Design review of the part built by this model. Coordinates are the model's own, in mm. A direction names the side the tool comes from. Coordinates: 2 decimals unless noted, no trailing zeros. Order: outer loops, then holes, each group sorted by start corner. A loop starts at its lowest first (then second) coordinate and runs counter-clockwise, first axis right, second up. Notation, with made-up numbers: M 41,54.5 L 59,54.5 A12 cw 59,63.5 Z; hole C 81,38 d1. An arc over 180 degrees is marked long. Answer in a Markdown table with one row per item.
Autodesk Fusion 360 part; units mm, degrees
sketch "Sketch1" plane through (0, 0, 0) normal (0, 1, 0) x (1, 0, 0)
  line L0 (55, -90) -> (-55, -90)
  line L1 (-55, -90) -> (-55, 90)
  line L2 (-55, 90) -> (55, 90)
  line L3 (55, 90) -> (55, -90)
  line L4 (55, -90) -> (-55, 90) construction
  line L5 (-55, -90) -> (55, 90) construction
  dimension "d1" = 180
  dimension "d2" = 110
extrude "Extrude1" add sketch "Sketch1" along normal blind 50
sketch "Sketch2" plane through (0, 50, 0) normal (0, 1, 0) x (-1, 0, 0)
  line L0 (-55, -90) -> (55, -90)
  line L1 (55, -90) -> (55, 90)
  line L2 (55, 90) -> (-55, 90)
  line L3 (-55, 90) -> (-55, -90)
  line L4 (55, -90) -> (30, -90)
  line L5 (30, -90) -> (30, -40)
  line L6 (30, -40) -> (55, -40)
  line L7 (55, -40) -> (55, -90)
  line L8 (30, -90) -> (10, -90)
  line L9 (10, -90) -> (10, -40)
  line L10 (10, -40) -> (30, -40)
  line L11 (30, -40) -> (30, -90)
  line L12 (10, -90) -> (-10, -90)
  line L13 (-10, -90) -> (-10, -40)
  line L14 (-10, -40) -> (10, -40)
  line L15 (10, -40) -> (10, -90)
  line L16 (-10, -90) -> (-30, -90)
  line L17 (-30, -90) -> (-30, -40)
  line L18 (-30, -40) -> (-10, -40)
  line L19 (-10, -40) -> (-10, -90)
  line L20 (-30, -90) -> (-55, -90)
  line L21 (-55, -90) -> (-55, -40)
  line L22 (-55, -40) -> (-30, -40)
  line L23 (-30, -40) -> (-30, -90)
  line L24 (55, 0) -> (-55, 0)
  line L25 (55, 90) -> (30, 90)
  line L26 (-10, 40) -> (10, 40)
  line L27 (-30, 40) -> (-30, 90)
  line L28 (-55, 90) -> (55, 90)
  line L29 (-30, 40) -> (-10, 40)
  line L30 (-30, 90) -> (-30, 40)
  line L31 (30, 90) -> (10, 90)
  line L32 (-10, 90) -> (-30, 90)
  line L33 (-55, 90) -> (-55, 40)
  line L34 (10, 40) -> (30, 40)
  line L35 (-10, 40) -> (-10, 90)
  line L36 (30, 90) -> (30, 40)
  line L37 (-55, 40) -> (-30, 40)
  line L38 (30, 40) -> (55, 40)
  line L39 (30, 40) -> (30, 90)
  line L40 (-30, 90) -> (-55, 90)
  line L41 (10, 40) -> (10, 90)
  line L42 (-10, 90) -> (-10, 40)
  line L43 (10, 90) -> (-10, 90)
  line L44 (10, 90) -> (10, 40)
  line L45 (55, 40) -> (55, 90)
  dimension "d5" = 25
  dimension "d6" = 50
  dimension "d7" = 20
  dimension "d8" = 20
  dimension "d9" = 20
  dimension "d10" = 25
  dimension "d11" = 50
  dimension "d12" = 50
  dimension "d13" = 50
  dimension "d14" = 50
  dimension "d15" = 110
extrude "Extrude2" cut sketch "Sketch2" against normal blind 50 contours L0 L13 L16 L17 L18 L19 L23 | L0 L5 L8 L9 L10 L11 L15 | L2 L27 L28 L29 L30 L32 L35 L42 | L2 L28 L31 L34 L36 L39 L41 L44
sketch "Sketch3" plane through (0, 50, 0) normal (0, 1, 0) x (-1, 0, 0)
  line L0 (-10, -40) -> (-10, -90)
  line L1 (-10, -90) -> (10, -90)
  line L2 (10, -90) -> (10, -40)
  line L3 (10, -40) -> (30, -40)
  line L4 (30, -40) -> (30, -90)
  line L5 (30, -90) -> (55, -90)
  line L6 (55, -90) -> (55, 90)
  line L7 (55, 90) -> (30, 90)
  line L8 (30, 90) -> (30, 40)
  line L9 (30, 40) -> (10, 40)
  line L10 (10, 40) -> (10, 90)
  line L11 (10, 90) -> (-10, 90)
  line L12 (-10, 90) -> (-10, 40)
  line L13 (-10, 40) -> (-30, 40)
  line L14 (-30, 40) -> (-30, 90)
  line L15 (-30, 90) -> (-55, 90)
  line L16 (-55, 90) -> (-55, -90)
  line L17 (-55, -90) -> (-30, -90)
  line L18 (-30, -90) -> (-30, -40)
  line L19 (-30, -40) -> (-10, -40)
hole "Hole1" at (0, 50, 0) direction (0, -1, 0) diameter 40 end through all
sketch "Sketch4" plane through (55, 0, 0) normal (1, 0, 0) x (0, 0, -1)
  line L0 (-90, 0) -> (90, 0)
  line L1 (90, 0) -> (90, 50)
  line L2 (90, 50) -> (-90, 50)
  line L3 (-90, 50) -> (-90, 0)
  circle A0 centre (65, 25) radius 25
  circle A1 centre (-65, 25) radius 25
  dimension "d21" = 50
  dimension "d23" = 50
  dimension "d24" = 65
  dimension "d25" = 25
  dimension "d26" = 25
  dimension "d27" = 65
extrude "Extrude3" cut sketch "Sketch4" against normal blind 110 contours L0 L3 A1 | L2 L3 A1 | L0 L1 A0 | L1 L2 A0
sketch "Sketch5" plane through (55, 0, 0) normal (1, 0, 0) x (0, 0, -1)
  arc A0 (-65, 50) -> (-65, 0) centre (-65, 25) ccw
  line L0 (-65, 0) -> (65, 0)
  arc A1 (65, 0) -> (65, 50) centre (65, 25) ccw
  line L1 (65, 50) -> (-65, 50)
  line L2 (-65, 25) -> (65, 25)
hole "Hole2" at (55, 25, 65) at (55, 25, -65) direction (-1, 0, 0) diameter 25 end through all
extrude "Extrude4" cut 1 faces at (55, 5.9862, 18.224) along direction (-1, 0, 0) blind 5
extrude "Extrude5" cut 1 faces at (-55, 5.9862, 18.224) along direction (1, 0, 0) blind 5
sketch "Sketch6" plane through (0, 50, 0) normal (0, 1, 0) x (-1, 0, 0)
  circle A0 centre (0, 0) radius 20
  line L0 (50, -65) -> (50, 65)
  line L1 (50, 65) -> (30, 65)
  line L2 (30, 65) -> (30, 40)
  line L3 (30, 40) -> (10, 40)
  line L4 (10, 40) -> (10, 65)
  line L5 (10, 65) -> (-10, 65)
  line L6 (-10, 65) -> (-10, 40)
  line L7 (-10, 40) -> (-30, 40)
  line L8 (-30, 40) -> (-30, 65)
  line L9 (-30, 65) -> (-50, 65)
  line L10 (-50, 65) -> (-50, -65)
  line L11 (-50, -65) -> (-30, -65)
  line L12 (-30, -65) -> (-30, -40)
  line L13 (-30, -40) -> (-10, -40)
  line L14 (-10, -40) -> (-10, -65)
  line L15 (-10, -65) -> (10, -65)
  line L16 (10, -65) -> (10, -40)
  line L17 (10, -40) -> (30, -40)
  line L18 (30, -40) -> (30, -65)
  line L19 (30, -65) -> (50, -65)
  line L20 (-50, -40) -> (50, -40)
  line L21 (50, -40) -> (50, 40)
  line L22 (50, 40) -> (-50, 40)
  line L23 (-50, 40) -> (-50, -40)
  line L24 (-50, -40) -> (50, 40) construction
  line L25 (50, -40) -> (-50, 40) construction
  dimension "d37" = 80
  dimension "d38" = 100
extrude "Extrude6" cut sketch "Sketch6" against normal blind 10 contours L0 L3 L7 L10 L13 L17 L20 L21 L22 L23
sketch "Sketch7" plane through (-50, 0, 0) normal (-1, 0, 0) x (0, 0, 1)
  line L0 (-40, 40) -> (-40, 50)
  line L1 (-40, 50) -> (-65, 50)
  arc A0 (-65, 50) -> (-65, 0) centre (-65, 25) ccw
  line L2 (-65, 0) -> (65, 0)
  arc A1 (65, 0) -> (65, 50) centre (65, 25) ccw
  line L3 (65, 50) -> (40, 50)
  line L4 (40, 50) -> (40, 40)
  line L5 (40, 40) -> (-40, 40)
  circle A2 centre (65, 25) radius 12.5
  circle A3 centre (-65, 25) radius 12.5
  circle A4 centre (-65, 25) radius 25
  circle A5 centre (65, 25) radius 25
  line L6 (-40, 40) -> (-45, 40)
  line L7 (40, 40) -> (45, 40)
extrude "Extrude7" cut sketch "Sketch7" against normal blind 100 contours L0 L1 A4 L6 | L3 L4 A5 L7
sketch "Sketch8" plane through (0, 0, 0) normal (0, -1, 0) x (1, 0, 0)
  line L0 (-50, 65) -> (-50, -65)
  line L1 (-50, -65) -> (-30, -65)
  line L2 (-30, -65) -> (-30, -40)
  line L3 (-30, -40) -> (-10, -40)
  line L4 (-10, -40) -> (-10, -65)
  line L5 (-10, -65) -> (10, -65)
  line L6 (10, -65) -> (10, -40)
  line L7 (10, -40) -> (30, -40)
  line L8 (30, -40) -> (30, -65)
  line L9 (30, -65) -> (50, -65)
  line L10 (50, -65) -> (50, 65)
  line L11 (50, 65) -> (30, 65)
  line L12 (30, 65) -> (30, 40)
  line L13 (30, 40) -> (10, 40)
  line L14 (10, 40) -> (10, 65)
  line L15 (10, 65) -> (-10, 65)
  line L16 (-10, 65) -> (-10, 40)
  line L17 (-10, 40) -> (-30, 40)
  line L18 (-30, 40) -> (-30, 65)
  line L19 (-30, 65) -> (-50, 65)
  circle A0 centre (0, 0) radius 20
  line L20 (50, 40) -> (-50, 40)
  line L21 (-50, 40) -> (-50, -40)
  line L22 (-50, -40) -> (50, -40)
  line L23 (50, -40) -> (50, 40)
  line L24 (50, 40) -> (-50, -40) construction
  line L25 (-50, 40) -> (50, -40) construction
  dimension "d43" = 80
extrude "Extrude8" cut sketch "Sketch8" against normal blind 10 contours L0 L3 L7 L10 L13 L17 L20 L21 L22 L23
sketch "Sketch9" plane through (-50, 0, 0) normal (-1, 0, 0) x (0, 0, 1)
  line L0 (40, 10) -> (40, 0)
  line L1 (40, 0) -> (65, 0)
  arc A0 (65, 0) -> (45, 40) centre (65, 25) ccw
  line L2 (45, 40) -> (-45, 40)
  arc A1 (-45, 40) -> (-65, 50) centre (-65, 25) ccw
  arc A2 (-65, 50) -> (-65, 0) centre (-65, 25) ccw
  line L3 (-65, 0) -> (-40, 0)
  line L4 (-40, 0) -> (-40, 10)
  line L5 (-40, 10) -> (40, 10)
  circle A3 centre (65, 25) radius 12.5
  circle A4 centre (-65, 25) radius 12.5
  circle A5 centre (-65, 25) radius 25
  circle A6 centre (65, 25) radius 25
  line L6 (-40, 10) -> (-45, 10)
  line L7 (40, 10) -> (45, 10)
  dimension "d46" = 50
extrude "Extrude9" cut sketch "Sketch9" against normal blind 100 contours L0 L1 A6 L7 | L3 L4 A5 L6
sketch "Sketch10" plane through (0, 40, 0) normal (0, 1, 0) x (-1, 0, 0)
  circle A0 centre (0, 0) radius 20
  line L0 (-50, 45) -> (-50, -45)
  line L1 (-50, -45) -> (-30, -45)
  line L2 (-30, -45) -> (-30, -40)
  line L3 (-30, -40) -> (-10, -40)
  line L4 (-10, -40) -> (-10, -45)
  line L5 (-10, -45) -> (10, -45)
  line L6 (10, -45) -> (10, -40)
  line L7 (10, -40) -> (30, -40)
  line L8 (30, -40) -> (30, -45)
  line L9 (30, -45) -> (50, -45)
  line L10 (50, -45) -> (50, 45)
  line L11 (50, 45) -> (30, 45)
  line L12 (30, 45) -> (30, 40)
  line L13 (30, 40) -> (10, 40)
  line L14 (10, 40) -> (10, 45)
  line L15 (10, 45) -> (-10, 45)
  line L16 (-10, 45) -> (-10, 40)
  line L17 (-10, 40) -> (-30, 40)
  line L18 (-30, 40) -> (-30, 45)
  line L19 (-30, 45) -> (-50, 45)
sketch "Sketch11" plane through (0, 50, 0) normal (0, 1, 0) x (-1, 0, 0)
  line L0 (23, -18.071) -> (23, 18.071)
  arc A0 (23, 18.071) -> (-23, 18.071) centre (0, 0) ccw
  line L1 (-23, 18.071) -> (-23, -18.071)
  arc A1 (-23, -18.071) -> (23, -18.071) centre (0, 0) ccw
  circle A2 centre (0, 0) radius 12
  circle A3 centre (12.5, 21.6506) radius 2.25
  circle A4 centre (12.5, -21.6506) radius 2.25
  circle A5 centre (-12.5, -21.6506) radius 2.25
  circle A6 centre (-12.5, 21.6506) radius 2.25
  circle A7 centre (12.5, 21.6506) radius 2.25
  circle A8 centre (12.5, -21.6506) radius 2.25
  circle A9 centre (-12.5, -21.6506) radius 2.25
  circle A10 centre (-12.5, 21.6506) radius 2.25
hole "Hole3" at (-12.5, 50, 21.6506) at (-12.5, 50, -21.6506) at (12.5, 50, 21.6506) at (12.5, 50, -21.6506) direction (0, -1, 0) diameter 3.332 depth 25 tip angle 118
(1) Add section A-A, the plane x = 0. Give the boundary of the cut face in (y, z), and give its area (3 significant figures).
Return value:
| item | result |
|---|---|
| outline | M 10,-45 A25 ccw long 40,-45 L 40,-20 L 10,-20 Z; M 10,20 L 40,20 L 40,45 A25 ccw long 10,45 Z; hole C 25,-65 d25; hole C 25,65 d25 |
| area | 4,240 mm2 |
(2) Draft analysis for pull direction Y (two halves, no side actions). For faces 4 (the flat face through (-20, 25, -40)), 5 (the cylindrical face through (39.86, 24.45, 77.488)), 6 (the flat face through (-12, 10, 19)), state which applies: pulls with the +Y half, pulls with the -Y half, needs draft (parallel to the pull), parting line crosses it, or undercut.
Return value:
| item | result |
|---|---|
| face 4 | needs draft |
| face 5 | undercut |
| face 6 | pulls with the -Y half |
(3) Insertion check: pin 1 Ø16 at (x, y) = (-23, 23.5) entering from +Z; pin 2 Ø12 at (x, z) = (-8.5, -32.5) entering from -Y; pin 3 Ø12 at (x, y) = (-29.5, 15) entering from +Z; pin 4 Ø20 at (y, z) = (25, -65) entering from +X. Each pin has a flat end and moves straight along its axis. Give the tip position at first contact, or say it passes through.
Return value:
| item | result |
|---|---|
| pin 1 | stops at z = 90 |
| pin 2 | stops at y = 10 |
| pin 3 | stops at z = 89.67 |
| pin 4 | passes through |
(4) Add section C-C, the plane z = 65. Give the boundary of the cut face in (x, y).
Return value:
| item | result |
|---|---|
| outline | M -50,0 L -30,0 L -30,12.5 L -50,12.5 Z; M -50,37.5 L -30,37.5 L -30,50 L -50,50 Z; M -10,0 L 10,0 L 10,12.5 L -10,12.5 Z; M -10,37.5 L 10,37.5 L 10,50 L -10,50 Z; M 30,0 L 50,0 L 50,12.5 L 30,12.5 Z; M 30,37.5 L 50,37.5 L 50,50 L 30,50 Z |
(5) For faces 1 (the cylindrical face through (14.126, 32.395, 21.289)), 2 (the flat face through (10, 40, 19)), 3 (the flat face through (20, 25, 40)), list the 3-axis set-ups (+Z, -Z, +X, -X, +Y, -Y) from which the entire face can be reached by the end or side of a thin tool; tool diameter is ignored.
Return value:
| item | result |
|---|---|
| face 1 | +Y |
| face 2 | +X, -X, +Y |
| face 3 | +Z, +Y, -Y |
(6) For line 1 along X through (y, z) = (16, 51); line 2 along Z through (x, y) = (-42, 25); line 3 along Y through (x, z) = (43.5, -65), list the stretches that pass through material, from the lowest coordinate up. Write a range as from..to.
Return value:
| item | result |
|---|---|
| line 1 | x = -50..-30, -10..10, 30..50 |
| line 2 | z = -90..-77.5, -52.5..52.5, 77.5..90 |
| line 3 | y = 0..12.5, 37.5..50 |
(7) Add section B-B, the plane z = 0. Give the boundary of the cut face in (x, y), and give its area (3 significant figures).
Return value:
| item | result |
|---|---|
| outline | M -50,10 L -20,10 L -20,40 L -50,40 Z; M 20,10 L 50,10 L 50,40 L 20,40 Z |
| area | 1,800 mm2 |
(8) Add section D-D, the plane x = -36. Give the boundary of the cut face in (y, z), and give its area (3 significant figures).
Return value:
| item | result |
|---|---|
| outline | M 10,-45 A25 ccw long 40,-45 L 40,45 A25 ccw long 10,45 Z; hole C 25,-65 d25; hole C 25,65 d25 |
| area | 5,440 mm2 |
